CAD build for the part. Positions are in the model's coordinates, mm. Face numbers are marked on the shaded views. A direction names the side the tool comes from. Round coordinates to 2 decimals unless told otherwise and drop trailing zeros. Loops run counter-clockwise (first coordinate to the right, second up) from the corner with the lowest first, then second, coordinate; pieces in that order, holes last. Notation, with made-up numbers: (-9.5, -35.5) -> (-0.5, -35.5) arc R23 cw to (-0.5, -25.5) -> close; hole circle Ø3 at (-7.5, 68.25). An arc over 180 degrees is marked (long way). Answer as CSV lines item,"result".
```python
from build123d import *

# Parameters (mm, degrees)
F1_DEPTH = 50
F2_R     = 10
F3_DEPTH = 61.142308
F4_R     = 20


with BuildPart() as f1:
    # F0 (on Front) → F1 (new body)
    with BuildSketch(Plane.XZ):
        Polygon((0, 39.717391), (0, 0), (61.141308, 0), (61.141308, 9.978262), (42.945653, 9.978262), (42.945653, 39.717391), (34.141306, 39.717391), (34.141306, 9.978262), (10.858696, 9.978262), (10.858696, 39.717391), align=None)
    extrude(amount=F1_DEPTH)

    # F2 (on face) → F3 (cut, through all)
    with BuildSketch(Plane(origin=(0, 0, 0), x_dir=(0, -1, 0), z_dir=(-1, 0, 0))):
        with Locations((25, 24.717391)):
            Circle(F2_R)
    extrude(amount=-F3_DEPTH, mode=Mode.SUBTRACT)

    # F4
    f4_edges = [f1.edges().sort_by_distance(p)[0] for p in [
        (61.141308, 0, 4.989131),
        (61.141308, -50, 4.989131),
    ]]
    fillet(f4_edges, radius=F4_R)


solid = f1.part
```
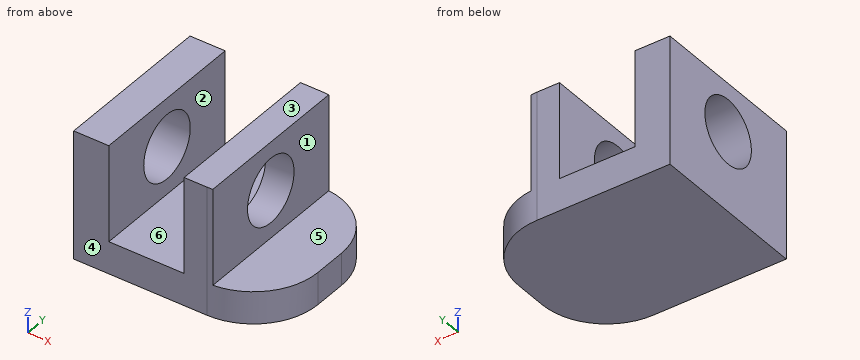
Q1. Two-plate mould, pull along X, no slides. Class the marked faces 1, 2 and 3: pulls with the +X half, pulls with the -X half, needs draft (parallel to the pull), parting line crosses it, or undercut.
Results:
face 1,"pulls with the +X half"
face 2,"undercut"
face 3,"needs draft"
Q2. Slice it at C-C, the plane z = 32. Give the cut face in (x, y).
Results:
outline,"(0, -50) -> (10.86, -50) -> (10.86, -31.85) -> (0, -31.85) -> close; (0, -18.15) -> (10.86, -18.15) -> (10.86, 0) -> (0, 0) -> close; (34.14, -50) -> (41.14, -50) arc R20 ccw to (42.95, -49.92) -> (42.95, -31.85) -> (34.14, -31.85) -> close; (34.14, -18.15) -> (42.95, -18.15) -> (42.95, -0.08) arc R20 ccw to (41.14, 0) -> (34.14, 0) -> close"
Q3. Drop flat-ended pins along their axis: pin 1 Ø16 at (y, z) = (-25, 24.72) entering from +X; pin 2 Ø4 at (y, z) = (-20.5, 10) entering from -X; pin 3 Ø10 at (y, z) = (-10, 29) entering from +X; pin 4 Ø9 at (x, y) = (48.5, -24) entering from +Z. Give the stop position or say it passes through.
Results:
pin 1,"through"
pin 2,"x = 0"
pin 3,"x = 42.95"
pin 4,"z = 9.98"
Q4. Slice it at A-A, the plane y = -25. Give the cut face in (x, z), and give its area (3 significant figures).
Results:
outline,"(0, 0) -> (61.14, 0) -> (61.14, 9.98) -> (42.95, 9.98) -> (42.95, 14.72) -> (34.14, 14.72) -> (34.14, 9.98) -> (10.86, 9.98) -> (10.86, 14.72) -> (0, 14.72) -> close; (0, 34.72) -> (10.86, 34.72) -> (10.86, 39.72) -> (0, 39.72) -> close; (34.14, 34.72) -> (42.95, 34.72) -> (42.95, 39.72) -> (34.14, 39.72) -> close"
area,"802 mm2"
Q5. Slice it at B-B, the plane z = 3. Give the cut face in (x, y), and give its area (3 significant figures).
Results:
outline,"(0, -50) -> (41.14, -50) arc R20 ccw to (61.14, -30) -> (61.14, -20) arc R20 ccw to (41.14, 0) -> (0, 0) -> close"
area,"2,890 mm2"
Q6. Slice it at D-D, the plane y = -36. Give the cut face in (x, z).
Results:
outline,"(0, 0) -> (60.22, 0) -> (60.22, 9.98) -> (42.95, 9.98) -> (42.95, 39.72) -> (34.14, 39.72) -> (34.14, 9.98) -> (10.86, 9.98) -> (10.86, 39.72) -> (0, 39.72) -> close"
Q7. Probe L1, parallel to Z at x = 8, y = -25; L2, parallel to X at y = -43, z = 19; L3, parallel to Z at x = 21, y = -47. List the from-to ranges inside material, lowest first. Write a range as [from, to].
Results:
L1,"[0, 14.72], [34.72, 39.72]"
L2,"[0, 10.86], [34.14, 42.95]"
L3,"[0, 9.98]"
Q8. Tool access for the marked faces 4, 5 and 6: list every direction of +Z, -Z, +X, -X, +Y, -Y with a clear straight run to the whole face (end or side of a thin tool).
Results:
face 4,"+Z, -Z, +X, -X, -Y"
face 5,"+Z, +X, +Y, -Y"
face 6,"+Z, +Y, -Y"
